Input: part model. Units: mm. Frame: model coordinates. Face numbers are marked on the shaded views. A direction names the side the tool comes from. Round coordinates to 2 decimals unless told otherwise and drop trailing zeros. Order: outer loops, then holes, each group sorted by start corner. A loop starts at its lowest first (then second) coordinate and runs counter-clockwise, first axis right, second up. Notation, with made-up numbers: (40, -13) -> (48, -13) arc R23 ccw to (48, 26) -> close; hole circle Ø11 at (61.5, 89). An arc over 180 degrees is marked (long way). Use a Markdown table: item, result.
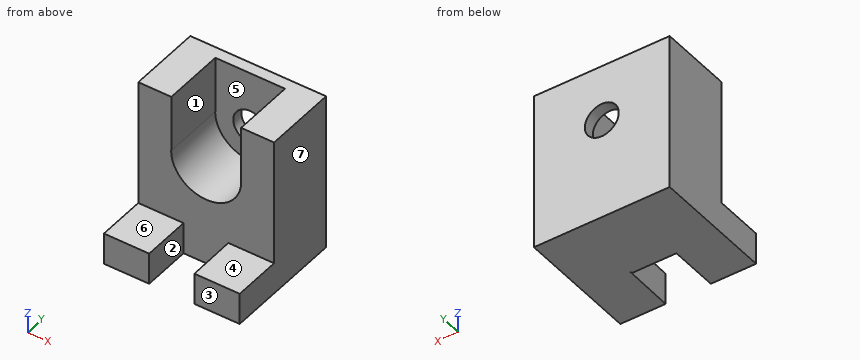
from build123d import *

# Parameters (mm, degrees)
F0_W      = 600
F0_H      = 700
F1_DEPTH  = 540
F2_W      = 600
F2_H      = 560
F3_DEPTH  = 240
F5_DEPTH  = 140.001
F7_DEPTH  = 25
F8_DEPTH  = 250
F9_R      = 75
F10_DEPTH = 50.001


with BuildPart() as f1:
    # F0 (on Front) → F1 (new body)
    with BuildSketch(Plane.XZ):
        Rectangle(F0_W, F0_H)
    extrude(amount=F1_DEPTH)

    # F2 (on face) → F3 (cut)
    with BuildSketch(Plane.XZ.offset(540)):
        with Locations((0, 70)):
            Rectangle(F2_W, F2_H)
    extrude(amount=-F3_DEPTH, mode=Mode.SUBTRACT)

    # F4 (on face) → F5 (cut, through all)
    with BuildSketch(Plane.XY.offset(-210)):
        Polygon((97.4877998233, -300), (-100, -300), (-100, -540), (100, -540), align=None)
    extrude(amount=-F5_DEPTH, mode=Mode.SUBTRACT)

    # F6 (on face) → F7 (join)
    with BuildSketch(Plane.XZ.offset(300)):
        with BuildLine():
            Line((154.0926195456, 100), (155, 100))
            ThreePointArc((155, 100), (0, -55), (-155, 100))
            Line((-155, 100), (-154.0926195456, 100))
            Line((-154.0926195456, 100), (-154.0926195456, 350))
            Line((-154.0926195456, 350), (-300, 350))
            Line((-300, 350), (-300, -210))
            Line((-300, -210), (-100, -210))
            Line((-100, -210), (-100, -350))
            Line((-100, -350), (97.4877998233, -350))
            Line((97.4877998233, -350), (97.4877998233, -210))
            Line((97.4877998233, -210), (300, -210))
            Line((300, -210), (300, 350))
            Line((300, 350), (154.0926195456, 350))
            Line((154.0926195456, 350), (154.0926195456, 100))
        make_face()
    extrude(amount=F7_DEPTH)

    # F8 (cut): faces of the model
    f8_faces = [f1.faces().sort_by_distance(p)[0] for p in [
        (0, -300, 162.2749017605),
        (0, -300, 162.2749017605),
    ]]
    extrude(f8_faces, amount=-F8_DEPTH, mode=Mode.SUBTRACT)

    # F9 (on face) → F10 (cut, through all)
    with BuildSketch(Plane.XZ.offset(50)):
        with Locations((0, 100)):
            Circle(F9_R)
    extrude(amount=-F10_DEPTH, mode=Mode.SUBTRACT)


solid = f1.part
1) Line query: L1, parallel to Z at x = 0, y = -15; L2, parallel to X at y = -96, z = 205; L3, parallel to Y at x = 167, z = 58. Output: solid intervals per line, ascending. Write a range as [from, to].
Results found:
| item | result |
|---|---|
| L1 | z = [-350, 25], [175, 350] |
| L2 | x = [-300, -154.09], [154.09, 300] |
| L3 | y = [-325, 0] |
2) Set-up query: the marked faces 1, 2, 3 and 4. Return all of +Z, -Z, +X, -X, +Y, -Y with unobstructed straight access to the full face (end or side cutting, diameter ignored); none if empty.
Results found:
| item | result |
|---|---|
| face 1 | +Z, -Y |
| face 2 | +Z, -Z, -Y |
| face 3 | +Z, -Z, +X, -X, -Y |
| face 4 | +Z, +X, -X, -Y |
3) Cut plane D-D on y = -443. Return loops of the section in (x, z), and give its area (3 significant figures).
Results found:
| item | result |
|---|---|
| outline | (-300, -350) -> (-100, -350) -> (-100, -210) -> (-300, -210) -> close; (98.98, -350) -> (300, -350) -> (300, -210) -> (98.98, -210) -> close |
| area | 56,100 mm² |
4) Pull-direction query (X, two-part tool) for the marked faces 5, 6 and 7; classes: +X half, -X half, draft (parallel to the pull), parting line (faces both ways), or undercut.
Results found:
| item | result |
|---|---|
| face 5 | undercut |
| face 6 | draft |
| face 7 | +X half |
5) Cut plane A-A on x = 0. Return loops of the section in (y, z), and give its area (3 significant figures).
Results found:
| item | result |
|---|---|
| outline | (-325, -350) -> (0, -350) -> (0, 25) -> (-50, 25) -> (-50, -55) -> (-325, -55) -> close; (-50, 175) -> (0, 175) -> (0, 350) -> (-50, 350) -> close |
| area | 109,000 mm² |
6) Cut plane C-C on y = -263. Return loops of the section in (x, z).
Results found:
| item | result |
|---|---|
| outline | (-300, -350) -> (300, -350) -> (300, 350) -> (154.09, 350) -> (154.09, 100) -> (155, 100) arc R155 cw to (-155, 100) -> (-154.09, 100) -> (-154.09, 350) -> (-300, 350) -> close |
7) Pin query (flat end, axial travel): pin 1 Ø3 at (x, z) = (1.5, -103) entering from +Y; pin 2 Ø6 at (x, z) = (-57.5, -136) entering from -Y; pin 3 Ø2 at (x, y) = (-167.5, -457.5) entering from +Z. Return the tip coordinate at first contact, or that it passes through.
Results found:
| item | result |
|---|---|
| pin 1 | stops at y = 0 |
| pin 2 | stops at y = -325 |
| pin 3 | stops at z = -210 |
8) Cut plane B-B on z = 280. Return loops of the section in (x, y), and give its area (3 significant figures).
Results found:
| item | result |
|---|---|
| outline | (-300, -325) -> (-154.09, -325) -> (-154.09, -50) -> (154.09, -50) -> (154.09, -325) -> (300, -325) -> (300, 0) -> (-300, 0) -> close |
| area | 110,000 mm² |
